```python
from build123d import *
from build123d import SkipClean  # not in build123d's __all__

# Parameters (mm, degrees)
F0_R     = 4
F1_DEPTH = 1
F2_W     = 15
F2_H     = 15
F2_R     = 5
F2_R_2   = 4
F3_DEPTH = 1
F4_R     = 3
F5_R     = 0.75
F6_DEPTH = 25


# Not quite as in the source:
# - after a boolean that leaves OpenCascade's solid faulty, fix() repairs it


with BuildPart() as f1:
    # F0 (on Top) → F1 (new body)
    with BuildSketch(Plane.XY):
        Circle(F0_R)
        with BuildLine():
            ThreePointArc((1.1922665017, 0.3755004513), (1.2354823202, 0.1899564067), (1.25, 0))
            ThreePointArc((1.25, 0), (1.2354823202, -0.1899564067), (1.1922665017, -0.3755004513))
            ThreePointArc((1.1922665017, -0.3755004513), (2.3070654164, -0.559829563), (2.817766953, -1.567766953))
            ThreePointArc((2.817766953, -1.567766953), (1.3778105463, -2.8032492732), (0.3755004513, -1.1922665017))
            ThreePointArc((0.3755004513, -1.1922665017), (0, -1.25), (-0.3755004513, -1.1922665017))
            ThreePointArc((-0.3755004513, -1.1922665017), (-0.3322846327, -1.3778105463), (-0.317766953, -1.567766953))
            ThreePointArc((-0.317766953, -1.567766953), (-2.5757043429, -2.3070654164), (-1.1922665017, -0.3755004513))
            ThreePointArc((-1.1922665017, -0.3755004513), (-1.25, 0), (-1.1922665017, 0.3755004513))
            ThreePointArc((-1.1922665017, 0.3755004513), (-2.5757043429, 2.3070654164), (-0.317766953, 1.567766953))
            ThreePointArc((-0.317766953, 1.567766953), (-0.3322846327, 1.3778105463), (-0.3755004513, 1.1922665017))
            ThreePointArc((-0.3755004513, 1.1922665017), (0, 1.25), (0.3755004513, 1.1922665017))
            ThreePointArc((0.3755004513, 1.1922665017), (1.3778105463, 2.8032492732), (2.817766953, 1.567766953))
            ThreePointArc((2.817766953, 1.567766953), (2.3070654164, 0.559829563), (1.1922665017, 0.3755004513))
        make_face(mode=Mode.SUBTRACT)
    extrude(amount=-F1_DEPTH)

    # F2 (on face) → F3 (join)
    with BuildSketch(Plane.XY):
        Rectangle(F2_W, F2_H)
        Circle(F2_R, mode=Mode.SUBTRACT)
        Circle(F2_R)
        Circle(F2_R_2, mode=Mode.SUBTRACT)
        Circle(F2_R_2)
        with BuildLine():
            ThreePointArc((1.1922665017, 0.3755004513), (1.2354823202, 0.1899564067), (1.25, 0))
            ThreePointArc((1.25, 0), (1.2354823202, -0.1899564067), (1.1922665017, -0.3755004513))
            ThreePointArc((1.1922665017, -0.3755004513), (2.4516504294, -2.4516504294), (0.3755004513, -1.1922665017))
            ThreePointArc((0.3755004513, -1.1922665017), (0, -1.25), (-0.3755004513, -1.1922665017))
            ThreePointArc((-0.3755004513, -1.1922665017), (-2.4516504294, -2.4516504294), (-1.1922665017, -0.3755004513))
            ThreePointArc((-1.1922665017, -0.3755004513), (-1.25, 0), (-1.1922665017, 0.3755004513))
            ThreePointArc((-1.1922665017, 0.3755004513), (-2.5757043429, 2.3070654164), (-0.317766953, 1.567766953))
            ThreePointArc((-0.317766953, 1.567766953), (-0.3322846327, 1.3778105463), (-0.3755004513, 1.1922665017))
            ThreePointArc((-0.3755004513, 1.1922665017), (0, 1.25), (0.3755004513, 1.1922665017))
            ThreePointArc((0.3755004513, 1.1922665017), (1.3778105463, 2.8032492732), (2.817766953, 1.567766953))
            ThreePointArc((2.817766953, 1.567766953), (2.3070654164, 0.559829563), (1.1922665017, 0.3755004513))
        make_face(mode=Mode.SUBTRACT)
    with SkipClean():  # cleaning this boolean's faces spoils the solid; the shape is the same uncleaned
        extrude(amount=F3_DEPTH)

    # F4
    f4_edges = [f1.edges().sort_by_distance(p)[0] for p in [
        (-7.5, -7.5, 0.5),
        (7.5, -7.5, 0.5),
        (-7.5, 7.5, 0.5),
        (7.5, 7.5, 0.5),
    ]]
    fillet(f4_edges, radius=F4_R)

    # F5 (on face) → F6 (cut)
    with BuildSketch(Plane(origin=(0, 0, 0), x_dir=(1, 0, 0), z_dir=(0, 0, -1))):
        with Locations((-4.5, 4.5)):
            Circle(F5_R)
        with Locations((-2.5, 4.5)):
            Circle(F5_R)
        with Locations((4.5, -4.5)):
            Circle(F5_R)
        with Locations((4.5, -2.5)):
            Circle(F5_R)
    extrude(amount=-F6_DEPTH, mode=Mode.SUBTRACT)

    add(f1.part.fix(), mode=Mode.REPLACE)


solid = f1.part
```
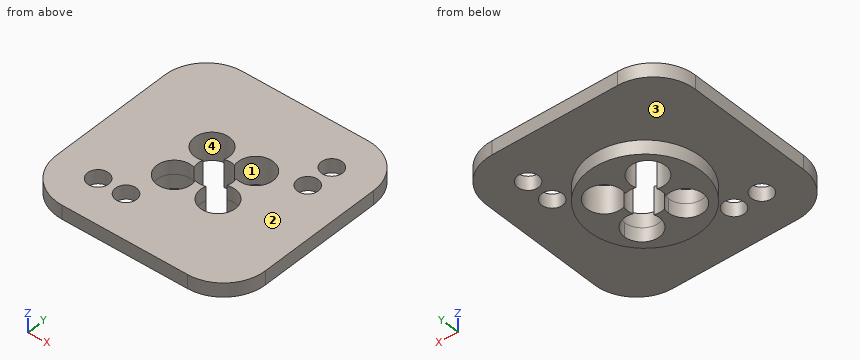
Can you work these out from the model? Positions are in its coordinate system, mm. Face numbers are marked on the shaded views. A direction names the side the tool comes from. Give positions to 0.01 mm unless a question says otherwise; leave off trailing zeros. Write each loop counter-clockwise with the first axis right and the second up, starting at its lowest first coordinate (ties: lowest second). Pieces come first, ordered by that corner, then holes. Notation, with made-up numbers: (18.5, 87) -> (44.5, 87) arc R15 cw to (44.5, 97) -> close; hole circle Ø5 at (80, 19.5). An arc over 180 degrees is marked (long way). One line per item, written item: value.
Q1. Imagine slicing it at D-D on y = 2.5. Please give me the cut outline in (x, z), and give its area (3 significant figures).
Results found:
outline: (-7.5, 0) -> (-3.12, 0) -> (-3.12, -1) -> (-2.4, -1) -> (-2.4, 1) -> (-7.5, 1) -> close; (-0.74, -1) -> (0.74, -1) -> (0.74, 1) -> (-0.74, 1) -> close; (2.4, -1) -> (3.12, -1) -> (3.12, 0) -> (3.75, 0) -> (3.75, 1) -> (2.4, 1) -> close; (5.25, 0) -> (7.5, 0) -> (7.5, 1) -> (5.25, 1) -> close
area: 13.1 mm^2
Q2. Imagine slicing it at A-A on x = 4.25. Please give me the cut outline in (y, z).
Results found:
outline: (-7.5, 0) -> (1.79, 0) -> (1.79, 1) -> (-7.5, 1) -> close; (3.21, 0) -> (3.79, 0) -> (3.79, 1) -> (3.21, 1) -> close; (5.21, 0) -> (7.5, 0) -> (7.5, 1) -> (5.21, 1) -> close
Q3. Please list where these lines run through material, in increasing order: line 1 (X direction, y = 1.5, z = 0.5); line 2 (Y direction, x = -4.5, z = 0.3); line 3 (X direction, y = 2.5, z = 0.95). Write a range as [from, to].
Results found:
line 1: x = [-7.5, -2.82], [-0.32, 0.32], [2.82, 7.5]
line 2: y = [-7.5, -5.25], [-3.75, 7.5]
line 3: x = [-7.5, -2.4], [-0.74, 0.74], [2.4, 3.75], [5.25, 7.5]
Q4. We'd pull the mould along X, two halves only. Please class the marked faces 1 and 2: +X half, -X half, draft (parallel to the pull), parting line (faces both ways), or undercut.
Results found:
face 1: undercut
face 2: draft
Q5. For P1, Ø1.4, axis at x = 4.5, y = 2.5, coming from the +Z side; P2, Ø1.7, axis at x = -4.5, y = -4.5, coming from the -Z side, each with a flat end and sliding along its axis, tell me the tip position at first contact or that it passes through.
Results found:
P1: passes through
P2: stops at z = 0
Q6. Which directions (+Z, -Z, +X, -X, +Y, -Y) give clear straight access to the entire face, cutting with the end or side of a thin tool? Please do the marked faces 3 and 4.
Results found:
face 3: -Z
face 4: +Z, -Z
Q7. Imagine slicing it at C-C on x = -2.5. Please give me the cut outline in (y, z).
Results found:
outline: (-7.5, 0) -> (-5.25, 0) -> (-5.25, 1) -> (-7.5, 1) -> close; (-3.75, 0) -> (-3.12, 0) -> (-3.12, -1) -> (-2.4, -1) -> (-2.4, 1) -> (-3.75, 1) -> close; (-0.74, -1) -> (0.74, -1) -> (0.74, 1) -> (-0.74, 1) -> close; (2.4, -1) -> (3.12, -1) -> (3.12, 0) -> (7.5, 0) -> (7.5, 1) -> (2.4, 1) -> close
Q8. Imagine slicing it at B-B on z = -0.7. Please give me the cut outline in (x, y).
Results found:
outline: circle Ø8 at (0, 0); hole (-1.19, -0.38) arc R1.25 ccw (long way) to (-0.38, -1.19) arc R1.25 ccw to (0.38, -1.19) arc R1.25 ccw (long way) to (1.19, -0.38) arc R1.25 ccw to (1.19, 0.38) arc R1.25 ccw (long way) to (0.38, 1.19) arc R1.25 ccw to (-0.38, 1.19) arc R1.25 ccw (long way) to (-1.19, 0.38) arc R1.25 ccw to start
